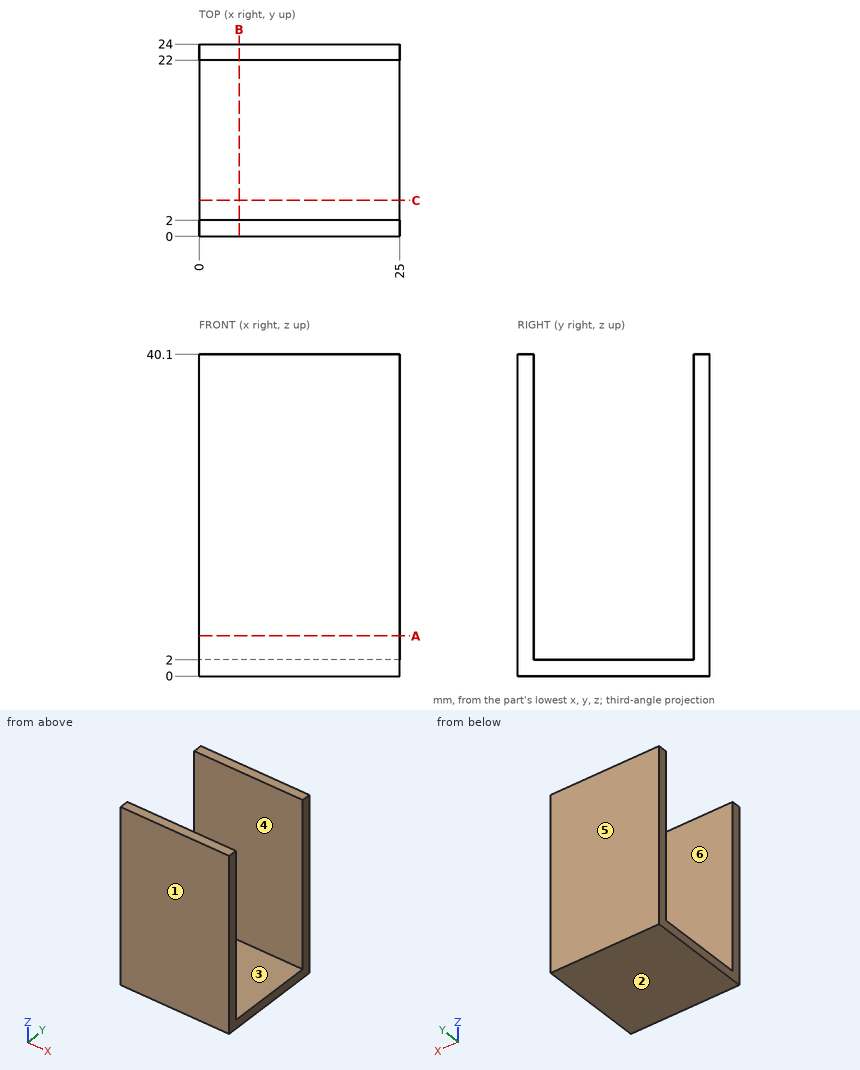
Check sheet for the drawn part. Datum: minimum x, y, z corner. Units: mm. A direction names the side the tool comes from. Give positions to 0.01 mm unless a question says otherwise; leave off trailing zeros. Loops run counter-clockwise (first coordinate to the right, second up) from the corner with the lowest first, then second, coordinate; pieces in that order, holes last.
1) Sectioned sample at B-B, the plane x = 5. Enter the section's corners in (y, z), then the cut area to 3 significant figures.
2) Sectioned sample at C-C, the plane y = 4.5. Enter the section's corners in (x, z).
3) Set-up check for the marked faces 5 and 6: record each of +Z, -Z, +X, -X, +Y, -Y from which the full face is reachable in a straight line by a thin tool's end or side.
4) Thickness scan on line 1 along Y through (x, z) = (14, 17.5); line 2 along Z through (x, y) = (16.5, 17.25). Record the ranges inside material, lowest first.
5) Sectioned sample at A-A, the plane z = 5. Enter the section's corners in (x, y).
6) Draft check along Y on the marked faces 1, 2, 3 and 4. Enter one of: pulls with the +Y half, pulls with the -Y half, needs draft (parallel to the pull), parting line crosses it, or undercut.
Answers:
1. outline: (0, 0) - (24, 0) - (24, 40.1) - (22, 40.1) - (22, 2) - (2, 2) - (2, 40.1) - (0, 40.1) - close
1. area: 200 mm2
2. outline: (0, 0) - (25, 0) - (25, 2) - (0, 2) - close
3. face 5: +Z, -Z, +X, -X, +Y
3. face 6: +Z, +X, -X
4. line 1: y = 0 to 2, 22 to 24
4. line 2: z = 0 to 2
5. outline: (0, 0) - (25, 0) - (25, 2) - (0, 2) - close; (0, 22) - (25, 22) - (25, 24) - (0, 24) - close
6. face 1: pulls with the -Y half
6. face 2: needs draft
6. face 3: undercut
6. face 4: undercut
